Input: part model. Units: mm. Frame: model coordinates. Face numbers are marked on the shaded views. Round coordinates to 2 decimals unless told otherwise and drop trailing zeros. Loops run counter-clockwise (first coordinate to the right, second up) from the corner with the lowest first, then second, coordinate; pieces in that order, holes last. Notation, with made-up numbers: (-25, 50) -> (-5, 50) arc R12 ccw to (-5, 68) -> close; hole circle Ø4 at (-27.5, -40). An arc over 180 degrees is marked (long way). Answer as a JSON object with one key per item and string values. Group by question number.
Item 1: Draft query along X for the marked faces 1, 2 and 3. Return one class per face: released by +X, released by -X, zero draft, split by the parting line, or undercut.
Item 2: Pin query (flat end, axial travel): pin 1 (6 mm diameter, centred on x = 38, z = 12.5, fed in from +Y). Return the tip coordinate at first contact, or that it passes through.
Item 3: Material intervals for line 1 (X direction, y = 5, z = 19); line 2 (Z direction, x = 21, y = 38.5); line 3 (X direction, y = 18.5, z = 11), sorted ascending. Write a range as [from, to].
Item 4: Section query A-A on y = 8.5. Return loops of the section in (x, z), and give its area (3 significant figures).
Item 5: Section query D-D on y = 35. Return loops of the section in (x, z).
Item 6: Section query C-C on z = -1. Return loops of the section in (x, y), and give its area (3 significant figures).
Item 7: Section query B-B on x = 38.5. Return loops of the section in (y, z).
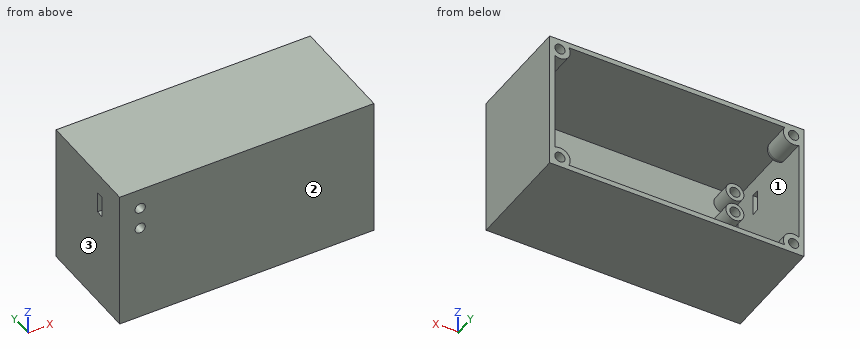
from build123d import *

# Parameters (mm, degrees)
SKETCH1_W           = 99
SKETCH1_H           = 54.5
BOSS_EXTRUDE1_DEPTH = 2
SKETCH2_W           = 99
SKETCH2_H           = 54.5
SKETCH2_W_2         = 95
SKETCH2_H_2         = 50.5
BOSS_EXTRUDE2_DEPTH = 40
SKETCH4_R           = 3.5
SKETCH4_R_2         = 2
BOSS_EXTRUDE3_DEPTH = 8
CUT_EXTRUDE1_START  = -2
SKETCH4_2_R         = 2
CUT_EXTRUDE1_DEPTH  = 2
SKETCH6_W           = 8.3
SKETCH6_H           = 3.1
CUT_EXTRUDE2_DEPTH  = 2
BOSS_EXTRUDE4_DEPTH = 12
SKETCH7_4_R         = 2
CUT_EXTRUDE3_DEPTH  = 10
FILLET1_R           = 2


with BuildPart() as part:
    # Sketch1 → Boss-Extrude1 (new body)
    with BuildSketch(Plane(origin=(0, 0, 0), x_dir=(1, 0, 0), z_dir=(0, 1, 0))):
        Rectangle(SKETCH1_W, SKETCH1_H)
    extrude(amount=BOSS_EXTRUDE1_DEPTH)

    # Sketch2 → Boss-Extrude2 (add)
    with BuildSketch(Plane(origin=(0, 2, 0), x_dir=(1, 0, 0), z_dir=(0, 1, 0))):
        Rectangle(SKETCH2_W, SKETCH2_H)
        Rectangle(SKETCH2_W_2, SKETCH2_H_2, mode=Mode.SUBTRACT)
    extrude(amount=BOSS_EXTRUDE2_DEPTH)

    # Sketch4 → Boss-Extrude3 (add)
    # profile 1 of 2: a face of its own
    with BuildSketch(Plane(origin=(0, 2, 0), x_dir=(1, 0, 0), z_dir=(0, 1, 0))):
        with Locations(Location((-41.5, -19.25, 0), (0, 0, 270))):
            Circle(SKETCH4_R)
        with Locations(Location((-41.5, -19.25, 0), (0, 0, 270))):
            Circle(SKETCH4_R_2, mode=Mode.SUBTRACT)
    # profile 2 of 2: a face of its own
    with BuildSketch(Plane(origin=(0, 2, 0), x_dir=(1, 0, 0), z_dir=(0, 1, 0))):
        with Locations(Location((-41.5, -10.75, 0), (0, 0, 270))):
            Circle(SKETCH4_R)
        with Locations(Location((-41.5, -10.75, 0), (0, 0, 270))):
            Circle(SKETCH4_R_2, mode=Mode.SUBTRACT)
    extrude(amount=BOSS_EXTRUDE3_DEPTH)

    # Sketch4<2> → Cut-Extrude1 (cut)
    with BuildSketch(Plane(origin=(0, 2, 0), x_dir=(1, 0, 0), z_dir=(0, 1, 0)).offset(CUT_EXTRUDE1_START)):
        with Locations(Location((-41.5, -10.75, 0), (0, 0, 270))):
            Circle(SKETCH4_2_R)
        with Locations(Location((-41.5, -19.25, 0), (0, 0, 270))):
            Circle(SKETCH4_2_R)
    extrude(amount=CUT_EXTRUDE1_DEPTH, mode=Mode.SUBTRACT)

    # Sketch6 → Cut-Extrude2 (cut)
    with BuildSketch(Plane(origin=(-47.5, 0, 0), x_dir=(0, 0, -1), z_dir=(1, 0, 0))):
        with Locations((-15, 13.15)):
            Rectangle(SKETCH6_W, SKETCH6_H)
    extrude(amount=-CUT_EXTRUDE2_DEPTH, mode=Mode.SUBTRACT)

    # Sketch7 → Boss-Extrude4 (add)
    with BuildSketch(Plane(origin=(0, 42, 0), x_dir=(1, 0, 0), z_dir=(0, 1, 0))):
        with BuildLine():
            ThreePointArc((-47.5, 19.785898385), (-42.671572875, 20.421572875), (-42.035898385, 25.25))
            Line((-42.035898385, 25.25), (-47.5, 25.25))
            Line((-47.5, 25.25), (-47.5, 19.785898385))
        make_face()
        with BuildLine():
            ThreePointArc((42.035898385, 25.25), (42.671572875, 20.421572875), (47.5, 19.785898385))
            Line((47.5, 19.785898385), (47.5, 25.25))
            Line((47.5, 25.25), (42.035898385, 25.25))
        make_face()
        with BuildLine():
            Line((47.5, -25.25), (47.5, -19.785898385))
            ThreePointArc((47.5, -19.785898385), (42.671572875, -20.421572875), (42.035898385, -25.25))
            Line((42.035898385, -25.25), (47.5, -25.25))
        make_face()
        with BuildLine():
            ThreePointArc((-42.035898385, -25.25), (-42.671572875, -20.421572875), (-47.5, -19.785898385))
            Line((-47.5, -19.785898385), (-47.5, -25.25))
            Line((-47.5, -25.25), (-42.035898385, -25.25))
        make_face()
    extrude(amount=-BOSS_EXTRUDE4_DEPTH)

    # Sketch7<4> → Cut-Extrude3 (cut)
    with BuildSketch(Plane(origin=(0, 42, 0), x_dir=(1, 0, 0), z_dir=(0, 1, 0))):
        with Locations(Location((-45.5, 23.25, 0), (0, 0, 270))):
            Circle(SKETCH7_4_R)
        with Locations(Location((45.5, 23.25, 0), (0, 0, 90))):
            Circle(SKETCH7_4_R)
        with Locations(Location((-45.5, -23.25, 0), (0, 0, 90))):
            Circle(SKETCH7_4_R)
        with Locations(Location((45.5, -23.25, 0), (0, 0, 270))):
            Circle(SKETCH7_4_R)
    extrude(amount=-CUT_EXTRUDE3_DEPTH, mode=Mode.SUBTRACT)

    # Fillet1
    fillet1_edges = [part.edges().sort_by_distance(p)[0] for p in [
        (42.671572875, 30, -20.421572875),
        (-42.671572875, 30, 20.421572875),
        (-42.671572875, 30, -20.421572875),
        (42.671572875, 30, 20.421572875),
    ]]
    fillet(fillet1_edges, radius=FILLET1_R - 0.0001)  # a hair under: the kernel refuses the full size


solid = part.part
Solved:
{
 "1": {"face 1": "undercut", "face 2": "zero draft", "face 3": "released by -X"},
 "2": {"pin 1": "y = 2"},
 "3": {"line 1": "[-49.5, -47.5], [-44.99, -43.48], [-39.52, -38.01], [47.5, 49.5]", "line 2": "[-27.25, -25.25], [25.25, 27.25]", "line 3": "[-49.5, -47.5], [47.5, 49.5]"},
 "4": {"outline": "(-49.5, -27.25) -> (49.5, -27.25) -> (49.5, 27.25) -> (-49.5, 27.25) -> close; circle Ø7 at (-41.5, 10.75); circle Ø7 at (-41.5, 19.25); hole (-47.5, -25.25) -> (47.5, -25.25) -> (47.5, 25.25) -> (-47.5, 25.25) -> close; hole circle Ø4 at (-41.5, 10.75); hole circle Ø4 at (-41.5, 19.25)", "area": "650 mm²"},
 "5": {"outline": "(-49.5, -27.25) -> (49.5, -27.25) -> (49.5, 27.25) -> (-49.5, 27.25) -> close; hole circle Ø4 at (-45.5, -23.25); hole (-47.5, -19.79) arc R4 cw to (-42.04, -25.25) -> (42.04, -25.25) arc R4 cw to (47.5, -19.79) -> (47.5, 19.79) arc R4 cw to (42.04, 25.25) -> (-42.04, 25.25) arc R4 cw to (-47.5, 19.79) -> close; hole circle Ø4 at (-45.5, 23.25); hole circle Ø4 at (45.5, -23.25); hole circle Ø4 at (45.5, 23.25)"},
 "6": {"outline": "(-49.5, 0) -> (49.5, 0) -> (49.5, 42) -> (47.5, 42) -> (47.5, 2) -> (-47.5, 2) -> (-47.5, 42) -> (-49.5, 42) -> close", "area": "358 mm²"},
 "7": {"outline": "(0, -27.25) -> (42, -27.25) -> (42, -25.25) -> (2, -25.25) -> (2, 25.25) -> (42, 25.25) -> (42, 27.25) -> (0, 27.25) -> close"}
}
